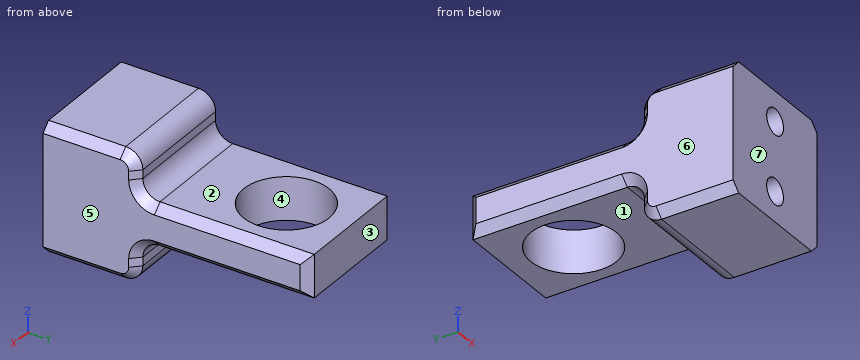
from build123d import *

# Parameters (mm, degrees)
SKETCH1_W           = 15
SKETCH1_H           = 15
BOSS_EXTRUDE1_DEPTH = 31
SKETCH2_R           = 5
CUT_EXTRUDE1_DEPTH  = 25
SKETCH3_W           = 15
SKETCH3_H           = 5
CUT_EXTRUDE2_DEPTH  = 20
FILLET4_R           = 2
CHAMFER1_SIZE       = 1
SKETCH4_R           = 1.5
CUT_EXTRUDE3_DEPTH  = 10


with BuildPart() as part:
    # Sketch1 → Boss-Extrude1 (new body)
    with BuildSketch(Plane(origin=(0, 0, 0), x_dir=(1, 0, 0), z_dir=(0, 1, 0))):
        Rectangle(SKETCH1_W, SKETCH1_H)
    extrude(amount=BOSS_EXTRUDE1_DEPTH)

    # Sketch2 → Cut-Extrude1 (cut)
    with BuildSketch(Plane.XY.offset(7.5)):
        with Locations((0, 23.5)):
            Circle(SKETCH2_R)
    extrude(amount=-CUT_EXTRUDE1_DEPTH, mode=Mode.SUBTRACT)

    # Sketch3 → Cut-Extrude2 (cut)
    with BuildSketch(Plane(origin=(0, 31, 0), x_dir=(1, 0, 0), z_dir=(0, 1, 0))):
        with Locations((0, 5)):
            Rectangle(SKETCH3_W, SKETCH3_H)
        with Locations((0, -5)):
            Rectangle(SKETCH3_W, SKETCH3_H)
    extrude(amount=-CUT_EXTRUDE2_DEPTH, mode=Mode.SUBTRACT)

    # Fillet4
    fillet4_edges = [part.edges().sort_by_distance(p)[0] for p in [
        (0, 11, -7.5),
        (0, 11, -2.5),
        (0, 11, 7.5),
        (0, 11, 2.5),
    ]]
    fillet(fillet4_edges, radius=FILLET4_R)

    # Chamfer1
    chamfer1_edges = [part.edges().sort_by_distance(p)[0] for p in [
        (-7.5, 31, 0),
        (7.5, 31, 0),
        (7.5, 11, 5),
        (-7.5, 11, 5),
        (7.5, 11, -5),
        (7.5, 22, -2.5),
        (7.5, 22, 2.5),
        (7.5, 4.5, 7.5),
        (7.5, 4.5, -7.5),
        (7.5, 10.414213562, -6.914213562),
        (7.5, 10.414213562, 6.914213562),
        (-7.5, 4.5, 7.5),
        (-7.5, 11, -5),
        (-7.5, 4.5, -7.5),
        (-7.5, 22, 2.5),
        (-7.5, 22, -2.5),
        (-7.5, 10.414213562, -6.914213562),
        (-7.5, 10.414213562, 6.914213562),
        (7.5, 11.585786438, -3.085786438),
        (-7.5, 11.585786438, -3.085786438),
        (-7.5, 11.585786438, 3.085786438),
        (7.5, 11.585786438, 3.085786438),
    ]]
    chamfer(chamfer1_edges, length=CHAMFER1_SIZE)

    # Sketch4 → Cut-Extrude3 (cut)
    with BuildSketch(Plane.XZ):
        with Locations(Location((0, 4, 0), (0, 0, 270))):
            Circle(SKETCH4_R)
        with Locations(Location((0, -4, 0), (0, 0, 270))):
            Circle(SKETCH4_R)
    extrude(amount=-CUT_EXTRUDE3_DEPTH, mode=Mode.SUBTRACT)


solid = part.part
Input: part model. Units: mm. Frame: model coordinates. Face numbers are marked on the shaded views. A direction names the side the tool comes from. Coordinates: 2 decimals unless noted, no trailing zeros. Order: outer loops, then holes, each group sorted by start corner. A loop starts at its lowest first (then second) coordinate and runs counter-clockwise, first axis right, second up. Notation, with made-up numbers: M 6,-38.75 L 65,-38.75 A21 cw 65,-0.75 Z; hole C -11.75,22.5 d3. An arc over 180 degrees is marked long. Answer as CSV lines item,"result".
1. Section B-B (y = 23.5). Return the cut outline in (x, z), then the cut area to 3 significant figures.
Reported:
outline,"M -7.5,-1.5 L -6.5,-2.5 L -5,-2.5 L -5,2.5 L -6.5,2.5 L -7.5,1.5 Z; M 5,-2.5 L 6.5,-2.5 L 7.5,-1.5 L 7.5,1.5 L 6.5,2.5 L 5,2.5 Z"
area,"23.0 mm2"
2. Section A-A (x = 4). Return the cut outline in (y, z).
Reported:
outline,"M 0,-7.5 L 9,-7.5 A2 ccw 11,-5.5 L 11,-4.5 A2 cw 13,-2.5 L 20.5,-2.5 L 20.5,2.5 L 13,2.5 A2 cw 11,4.5 L 11,5.5 A2 ccw 9,7.5 L 0,7.5 Z; M 26.5,-2.5 L 31,-2.5 L 31,2.5 L 26.5,2.5 Z"
3. Pull-direction query (X, two-part tool) for the marked faces 4, 5, 6 and 7; classes: released by +X, released by -X, zero draft, split by the parting line, or undercut.
Reported:
face 4,"undercut"
face 5,"released by +X"
face 6,"released by -X"
face 7,"zero draft"
4. Material intervals for line 1 (X direction, y = 6.75, z = 4); line 2 (Y direction, x = 0, z = 1.35); line 3 (Z direction, x = 0.75, y = 17), sorted ascending. Write a range as from..to.
Reported:
line 1,"-7.5..-1.5, 1.5..7.5"
line 2,"0..18.5, 28.5..31"
line 3,"-2.5..2.5"
5. Section C-C (z = -1). Return the cut outline in (x, y), then the cut area to 3 significant figures.
Reported:
outline,"M -7.5,0 L 7.5,0 L 7.5,30 L 6.5,31 L -6.5,31 L -7.5,30 Z; hole C 0,23.5 d10"
area,"385 mm2"
6. First-contact query: P1, Ø4, axis at y = 16, z = -5, coming from the -X side; P2, Ø0.9, axis at x = 0, z = -4.5, coming from the -Y side; P3, Ø6, axis at x = 2, y = 24, coming from the -Z side; P4, Ø2.5, axis at x = 0, z = 4, coming from the +Y side. Flat tips, straight axial feed; report the tip coordinate or a pass-through.
Reported:
P1,"through"
P2,"y = 10"
P3,"z = -2.5"
P4,"y = 12.03"
7. Access query for the marked faces 1, 2 and 3. Directions: +Z, -Z, +X, -X, +Y, -Y. A direction counts if a zero-diameter tool reaches every point of the face in a straight line with its end or side. Return the directions, or none.
Reported:
face 1,"-Z, +X, -X, +Y"
face 2,"+Z, +X, -X, +Y"
face 3,"+Z, -Z, +X, -X, +Y"
8. Section D-D (y = 4). Return the cut outline in (x, z).
Reported:
outline,"M -7.5,-6.5 L -6.5,-7.5 L 6.5,-7.5 L 7.5,-6.5 L 7.5,6.5 L 6.5,7.5 L -6.5,7.5 L -7.5,6.5 Z; hole C 0,-4 d3; hole C 0,4 d3"
